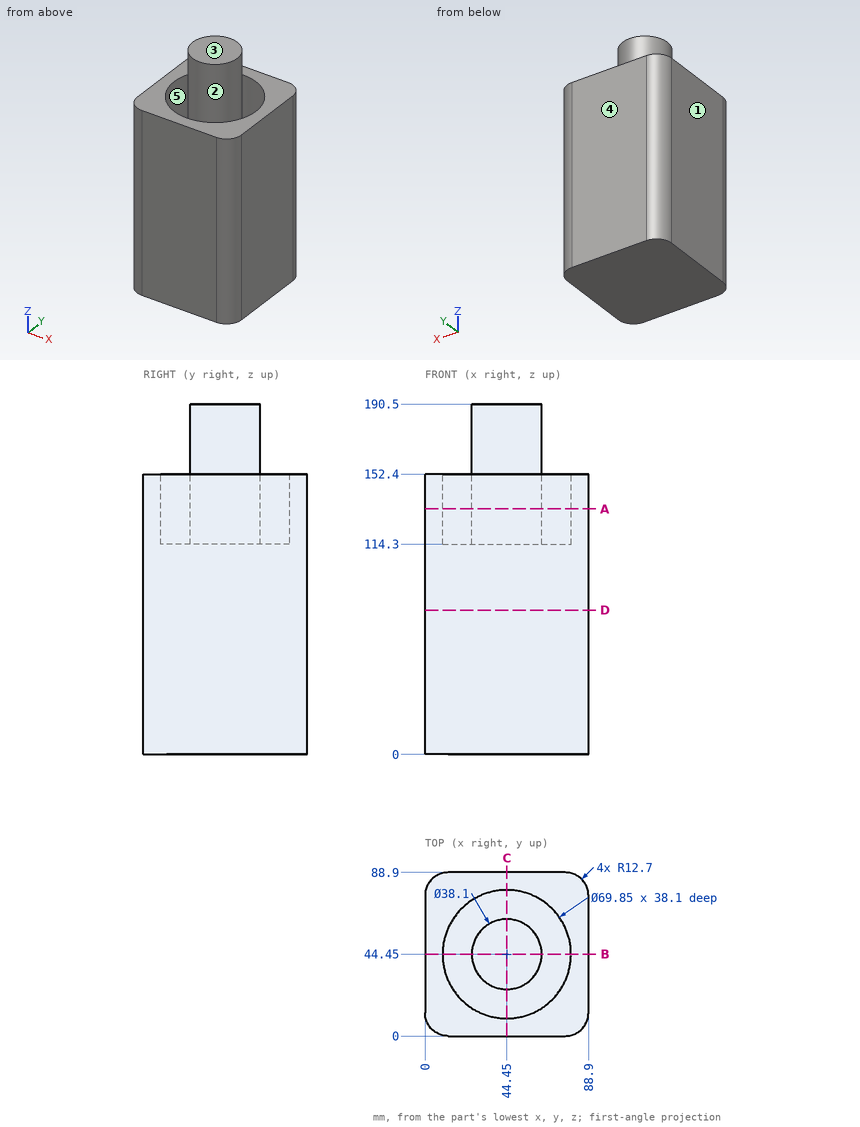
Job drawing, mm, ordinate dimensions from the low corner. One solid piece. A direction names the side the tool comes from. Round coordinates to 2 decimals unless told otherwise and drop trailing zeros. Write each loop counter-clockwise with the first axis right and the second up, starting at its lowest first coordinate (ties: lowest second). Pieces come first, ordered by that corner, then holes.
1) 3-axis set-ups, long thin cutter, end or side, ignore diameter. For the marked faces 1 and 2: which of +Z, -Z, +X, -X, +Y, -Y reach the whole face in a straight line?
2) Drill centre lines: probe 1 along Y at (x, z) = (44.45, 142) (3 decimals); probe 2 along Y at (x, z) = (49, 118). Where is each one in solid material? Low to high.
3) Band-saw the part on A-A, the plane z = 133.5. List the corners of the cut face in (x, y) (3 decimals), and give its area (3 significant figures).
4) Band-saw the part on D-D, the plane z = 78.5. List the corners of the cut face in (x, y), and give its area (3 significant figures).
5) Mould opens along Y. For the marked faces 3, 4 and 5 say: +Y half, -Y half, draft (parallel to the pull), parting line (faces both ways), or undercut.
6) Pin check, flat tips, straight feed: pin 1 (12 mm diameter, centred on y = 76.5, z = 45.5, fed in from +X); pin 2 (1.5 mm diameter, centred on y = 39, z = 157.5, fed in from -X); pin 3 (10 mm diameter, centred on x = 66.5, z = 170, fed in from -Y). Stop position of each tip, or through.
7) Band-saw the part on B-B, the plane y = 44.45. List the corners of the cut face in (x, z) (3 decimals).
Ans:
1. face 1: +Z, -Z, -X, +Y, -Y
1. face 2: +Z
2. probe 1: y = 0 to 9.525, 25.4 to 63.5, 79.375 to 88.9
2. probe 2: y = 0 to 9.82, 25.95 to 62.95, 79.08 to 88.9
3. outline: (0, 12.7) arc R12.7 ccw to (12.7, 0) - (76.2, 0) arc R12.7 ccw to (88.9, 12.7) - (88.9, 76.2) arc R12.7 ccw to (76.2, 88.9) - (12.7, 88.9) arc R12.7 ccw to (0, 76.2) - close; circle Ø38.1 at (44.45, 44.45); hole circle Ø69.85 at (44.45, 44.45)
3. area: 5,070 mm2
4. outline: (0, 12.7) arc R12.7 ccw to (12.7, 0) - (76.2, 0) arc R12.7 ccw to (88.9, 12.7) - (88.9, 76.2) arc R12.7 ccw to (76.2, 88.9) - (12.7, 88.9) arc R12.7 ccw to (0, 76.2) - close
4. area: 7,760 mm2
5. face 3: draft
5. face 4: +Y half
5. face 5: undercut
6. pin 1: stops at x = 88.9
6. pin 2: stops at x = 25.99
6. pin 3: stops at y = 35.95
7. outline: (0, 0) - (88.9, 0) - (88.9, 152.4) - (79.375, 152.4) - (79.375, 114.3) - (63.5, 114.3) - (63.5, 190.5) - (25.4, 190.5) - (25.4, 114.3) - (9.525, 114.3) - (9.525, 152.4) - (0, 152.4) - close
